Could you check a few things on this model? Use its own coordinates, in mm. A direction names the side the tool comes from. Give positions to 0.01 mm unless a question says otherwise; leave off trailing zeros. Order: outer loops, then holes, each group sorted by start corner. A loop starts at its lowest first (then second) coordinate and runs counter-clockwise, first axis right, second up. Notation, with made-up numbers: (-36, 19.5) - (9, 19.5) arc R23 ccw to (9, 50.5) - close; hole circle Ø11 at (-27.75, 83.5). An arc over 180 degrees is marked (long way). One line per question, with ' | ' between items. Start each with the question number.
1. For P1, Ø2, axis at y = 34, z = 0.5, coming from the +X side; P2, Ø2.5, axis at x = -45, y = 58, coming from the +Z side; P3, Ø8, axis at y = 68.5, z = -41, coming from the +X side, each with a flat end and sliding along its axis, tell me the tip position at first contact or that it passes through.
2. Which directions (+Z, -Z, +X, -X, +Y, -Y) give clear straight access to the entire face, cutting with the end or side of a thin tool? Please do faces 1 (the flat face through (37.06, 34.82, 27.87)), 2 (the flat face through (-50.707, 20, 1)), 3 (the flat face through (50.245, 58, 28)), 4 (the cylindrical face through (-45.593, 5.437, 11.512)).
3. I need wall thicknesses on probe 1 along Z at (x, y) = (31.5, 28); probe 2 along Z at (x, y) = (-44, 79); probe 3 along X at (y, z) = (53.5, 15). Which ranges of each line are inside material? Lowest first, please. Write a range as from..to.
4. If we mould it in two halves opening along Z, with no side actions, what happens to faces 5 (the flat face through (14, 18, -39.238)), 6 (the flat face through (-41.476, 116, 4)), 7 (the flat face through (14, 18, 40.238))? For each: released by +Z, released by -Z, zero draft, split by the parting line, or undercut.
5. Imagine slicing it at C-C (z = -44.5). Please give me the cut outline in (x, y), and give its area (3 significant figures).
6. Imagine slicing it at D-D (x = -18.5). Please give me the cut outline in (y, z).
7. Imagine slicing it at A-A (z = 37). Please give me the cut outline in (x, y), and give its area (3 significant figures).
8. Imagine slicing it at B-B (y = 76.5). Please give me the cut outline in (x, z).
```python
from build123d import *

# Parameters (mm, degrees)
SKETCH_1_W          = 120
SKETCH_1_H          = 110
EXTRUDE_1_DEPTH     = 120
SKETCH_2_W          = 119
SKETCH_2_H          = 119
CUT_EXTRUDE_1_DEPTH = 109
SKETCH_3_W          = 13.76951007
SKETCH_3_H          = 41.816324506
EXTRUDE_2_DEPTH     = 29
SKETCH_3_2_W        = 13.76951007
SKETCH_3_2_H        = 41.816324506
CUT_EXTRUDE_2_DEPTH = 9
SKETCH_6_R          = 1.856942382
EXTRUDE_4_DEPTH     = 9
SKETCH_7_W          = 6
SKETCH_7_H          = 27
EXTRUDE_5_DEPTH     = 2
SKETCH_8_W          = 2
SKETCH_8_H          = 2
EXTRUDE_6_DEPTH     = 3
SKETCH_9_W          = 4.691076501
SKETCH_9_H          = 101.472246916
EXTRUDE_7_DEPTH     = 83
SKETCH_10_W         = 95.77595166
SKETCH_10_H         = 78.098220696
CUT_EXTRUDE_3_DEPTH = 1
SKETCH_11_W         = 71.699562075
SKETCH_11_H         = 25.094846726
EXTRUDE_9_DEPTH     = 61
CUT_EXTRUDE_4_DEPTH = 81
SKETCH_13_R         = 1.5
EXTRUDE_10_DEPTH    = 31
SKETCH_14_W         = 23
SKETCH_14_H         = 14
EXTRUDE_11_DEPTH    = 2
SKETCH_15_W         = 21.829901038
SKETCH_15_H         = 12.722773114
CUT_EXTRUDE_5_DEPTH = 1


with BuildPart() as part:
    # Sketch 1 → Extrude 1 (new body)
    with BuildSketch(Plane(origin=(0, 0, 0), x_dir=(1, 0, 0), z_dir=(0, 1, 0))):
        Rectangle(SKETCH_1_W, SKETCH_1_H)
    extrude(amount=EXTRUDE_1_DEPTH)

    # Sketch 2 → Cut-Extrude 1 (cut)
    with BuildSketch(Plane.XY.offset(55)):
        with Locations((0.5, 60.5)):
            Rectangle(SKETCH_2_W, SKETCH_2_H)
    extrude(amount=-CUT_EXTRUDE_1_DEPTH, mode=Mode.SUBTRACT)

    # Sketch 3 → Extrude 2 (add)
    with BuildSketch(Plane(origin=(0, 1, 0), x_dir=(1, 0, 0), z_dir=(0, 1, 0))):
        with Locations((-43.822012207, -0.5)):
            Rectangle(SKETCH_3_W, SKETCH_3_H)
    extrude(amount=EXTRUDE_2_DEPTH)

    # Sketch 3_2 → Cut-Extrude 2 (cut)
    with BuildSketch(Plane(origin=(0, 1, 0), x_dir=(1, 0, 0), z_dir=(0, 1, 0))):
        with Locations((-43.822012207, -0.5)):
            Rectangle(SKETCH_3_2_W, SKETCH_3_2_H)
    extrude(amount=CUT_EXTRUDE_2_DEPTH, mode=Mode.SUBTRACT)


with BuildPart() as cut_extrude_2_piece_1:
    # of the separate pieces the step leaves, piece 1, a body of its own (cut_extrude_2_pieces)
    add(part.part.solids().sort_by_distance((-60, 0, -55))[0])



with BuildPart() as cut_extrude_2_piece_2:
    # of the separate pieces the step leaves, piece 2, a body of its own (cut_extrude_2_pieces)
    add(part.part.solids().sort_by_distance((-50.706767242, 10, -20.408162253))[0])


with BuildPart() as cut_extrude_2_piece_1_1:
    add(cut_extrude_2_piece_1.part)

    add(cut_extrude_2_piece_2.part)  # Extrude 4 merges Cut-Extrude 2 piece 2
    # Sketch 6 → Extrude 4 (add)
    with BuildSketch(Plane(origin=(0, 1, 0), x_dir=(1, 0, 0), z_dir=(0, 1, 0))):
        with Locations(Location((-43.822012207, -10.954081127, 0), (0, 0, 180))):
            Circle(SKETCH_6_R)
        with Locations((-43.822012207, 9.954081127)):
            Circle(SKETCH_6_R)
    extrude(amount=EXTRUDE_4_DEPTH)



with BuildPart() as body_2:
    # Sketch 7 → Extrude 5 (new body)
    with BuildSketch(Plane(origin=(0, 30, 0), x_dir=(1, 0, 0), z_dir=(0, 1, 0))):
        with Locations((-43.822012207, -0.5)):
            Rectangle(SKETCH_7_W, SKETCH_7_H)
    extrude(amount=EXTRUDE_5_DEPTH)


with BuildPart() as cut_extrude_2_piece_1_2:
    add(cut_extrude_2_piece_1_1.part)

    add(body_2.part)  # Extrude 6 merges body 2
    # Sketch 8 → Extrude 6 (add)
    with BuildSketch(Plane(origin=(0, 32, 0), x_dir=(1, 0, 0), z_dir=(0, 1, 0))):
        with Locations((-43.822012207, -0.5)):
            Rectangle(SKETCH_8_W, SKETCH_8_H)
    extrude(amount=EXTRUDE_6_DEPTH)

    # Sketch 9 → Extrude 7 (add)
    with BuildSketch(Plane(origin=(0, 35, 0), x_dir=(1, 0, 0), z_dir=(0, 1, 0))):
        with Locations((-43.822012208, -0.5)):
            Rectangle(SKETCH_9_W, SKETCH_9_H)
    extrude(amount=EXTRUDE_7_DEPTH)

    # Sketch 10 → Cut-Extrude 3 (cut)
    with BuildSketch(Plane(origin=(-41.476473957, 0, 0), x_dir=(0, 0, -1), z_dir=(1, 0, 0))):
        with Locations((-0.5, 76.5)):
            Rectangle(SKETCH_10_W, SKETCH_10_H)
    extrude(amount=-CUT_EXTRUDE_3_DEPTH, mode=Mode.SUBTRACT)

    # Sketch 11 → Extrude 9 (add)
    with BuildSketch(Plane(origin=(0, 1, 0), x_dir=(1, 0, 0), z_dir=(0, 1, 0))):
        with Locations((14.395545437, -27.691005805)):
            Rectangle(SKETCH_11_W, SKETCH_11_H)
        with Locations((14.395545437, 26.691005805)):
            Rectangle(SKETCH_11_W, SKETCH_11_H)
    extrude(amount=EXTRUDE_9_DEPTH)

    # Sketch 12 → Cut-Extrude 4 (cut)
    with BuildSketch(Plane.XY.offset(40.238429168)):
        Polygon((-3.329674483, 22.725113556), (23.497466254, 22.725113556), (50.245326474, 62), (-21.454235601, 62), (-21.454235601, 1), align=None)
        Polygon((23.497466254, 14.908243333), (23.497466254, 1), (50.245326474, 1), (50.245326474, 54.183129777), align=None)
        Polygon((-3.329674483, 14.908243333), (-14.932873043, 1), (-3.329674483, 1), align=None)
    extrude(amount=-CUT_EXTRUDE_4_DEPTH, mode=Mode.SUBTRACT)

    # Sketch 13 → Extrude 10 (add)
    with BuildSketch(Plane(origin=(0, 1, 0), x_dir=(1, 0, 0), z_dir=(0, 1, 0))):
        with Locations((0.5, -0.5)):
            Circle(SKETCH_13_R)
    extrude(amount=EXTRUDE_10_DEPTH)

    # Sketch 14 → Extrude 11 (add)
    with BuildSketch(Plane(origin=(0, 32, 0), x_dir=(1, 0, 0), z_dir=(0, 1, 0))):
        with Locations((0.5, -0.5)):
            Rectangle(SKETCH_14_W, SKETCH_14_H)
    extrude(amount=EXTRUDE_11_DEPTH)

    # Sketch 15 → Cut-Extrude 5 (cut)
    with BuildSketch(Plane(origin=(0, 34, 0), x_dir=(1, 0, 0), z_dir=(0, 1, 0))):
        with Locations((0.5, -0.5)):
            Rectangle(SKETCH_15_W, SKETCH_15_H)
    extrude(amount=-CUT_EXTRUDE_5_DEPTH, mode=Mode.SUBTRACT)


solid = cut_extrude_2_piece_1_2.part
```
Results found:
1) P1: stops at x = 12 | P2: stops at z = 51.24 | P3: stops at x = -42.48
2) face 1: +Z, +X | face 2: +Z, +Y | face 3: +Z, +X, +Y | face 4: none
3) probe 1: z = -55..-54, -39.24..-14.14, 15.14..40.24 | probe 2: z = -55..-54, -50.24..51.24 | probe 3: x = -60..-59, -46.17..-42.48
4) face 5: undercut | face 6: zero draft | face 7: released by +Z
5) outline: (-60, 0) - (60, 0) - (60, 1) - (-59, 1) - (-59, 120) - (-60, 120) - close; (-46.17, 35) - (-41.48, 35) - (-41.48, 37.45) - (-42.48, 37.45) - (-42.48, 115.55) - (-41.48, 115.55) - (-41.48, 118) - (-46.17, 118) - close | area: 550 mm2
6) outline: (0, -55) - (120, -55) - (120, -54) - (1, -54) - (1, -39.24) - (4.54, -39.24) - (4.54, -14.14) - (1, -14.14) - (1, 15.14) - (4.54, 15.14) - (4.54, 40.24) - (1, 40.24) - (1, 55) - (0, 55) - close
7) outline: (-60, 0) - (60, 0) - (60, 1) - (23.5, 1) - (23.5, 14.91) - (50.25, 54.18) - (50.25, 62) - (23.5, 22.73) - (-3.33, 22.73) - (-21.45, 1) - (-59, 1) - (-59, 120) - (-60, 120) - close; (-46.17, 35) - (-41.48, 35) - (-41.48, 37.45) - (-42.48, 37.45) - (-42.48, 115.55) - (-41.48, 115.55) - (-41.48, 118) - (-46.17, 118) - close; hole (-14.93, 1) - (-3.33, 1) - (-3.33, 14.91) - close | area: 1,460 mm2
8) outline: (-60, -55) - (60, -55) - (60, -54) - (-59, -54) - (-59, 55) - (-60, 55) - close; (-46.17, -50.24) - (-41.48, -50.24) - (-41.48, -47.39) - (-42.48, -47.39) - (-42.48, 48.39) - (-41.48, 48.39) - (-41.48, 51.24) - (-46.17, 51.24) - close
